from build123d import *

# Parameters (mm, degrees)
F0_R      = 4.925
F1_DEPTH  = 1.55
F2_W      = 1.55
F2_H      = 68.6
F3_DEPTH  = 16
F4_W      = 47.8
F4_H      = 1.55
F5_DEPTH  = 1.55
F6_W      = 47.8
F6_H      = 1.55
F7_DEPTH  = 34.2
F8_R      = 1.5
F10_DEPTH = 1.551


with BuildPart() as f1:
    # F0 (on Top) → F1 (new body)
    with BuildSketch(Plane.XY):
        Polygon((-51.3558513849, 10.4234758295), (-51.3558513849, -58.2765241705), (2.4441486151, -58.2765241705), (2.4441486151, -29.3765241705), (-37.3558513849, 10.4234758295), align=None)
        with BuildLine():
            ThreePointArc((-27.6816260073, -49.4227633754), (-35.7418681063, -49.3109720316), (-35.6300767624, -41.2507299325))
            Line((-35.6300767624, -41.2507299325), (-20.1462239232, -26.190507449))
            ThreePointArc((-20.1462239232, -26.190507449), (-13.9542389387, -25.0256630672), (-10.4719985456, -30.2765241705))
            ThreePointArc((-10.4719985456, -30.2765241705), (-10.9211374423, -32.4942837773), (-12.197773168, -34.3625408919))
            Line((-12.197773168, -34.3625408919), (-27.6816260073, -49.4227633754))
        make_face(mode=Mode.SUBTRACT)
        with Locations((-31.2308513849, -20.5015241705)):
            Circle(F0_R, mode=Mode.SUBTRACT)
    extrude(amount=F1_DEPTH)

    # F2 (on face) → F3 (join)
    with BuildSketch(Plane(origin=(0, 0, 0), x_dir=(1, 0, 0), z_dir=(0, 0, -1))):
        with Locations((-50.5808513849, 23.8765241705)):
            Rectangle(F2_W, F2_H)
    extrude(amount=F3_DEPTH)

    # F4 (on face) → F5 (join)
    with BuildSketch(Plane.XY.offset(1.55)):
        with Locations((-21.4558513849, -59.0515241705)):
            Rectangle(F4_W, F4_H)
    extrude(amount=-F5_DEPTH)

    # F6 (on face) → F7 (join)
    with BuildSketch(Plane.XY.offset(1.55)):
        with Locations((-21.4558513849, -59.0515241705)):
            Rectangle(F6_W, F6_H)
    extrude(amount=F7_DEPTH)

    # F8
    f8_edges = [f1.edges().sort_by_distance(p)[0] for p in [
        (-21.455851, -59.826524, 0),
        (-51.355851, -23.926524, 1.55),
    ]]
    fillet(f8_edges, radius=F8_R)

    # F9 (on face) → F10 (cut, through all)
    with BuildSketch(Plane(origin=(0, -58.2765241705, 0), x_dir=(-1, 0, 0), z_dir=(0, 1, 0))):
        with BuildLine():
            ThreePointArc((15.4058513849, 15.85), (19.3302940204, 17.4755573644), (20.9558513849, 21.4))
            ThreePointArc((20.9558513849, 21.4), (19.3302940204, 25.3244426356), (15.4058513849, 26.95))
            ThreePointArc((15.4058513849, 26.95), (9.8558513849, 21.4), (15.4058513849, 15.85))
        make_face()
        with BuildLine():
            ThreePointArc((15.4058513849, 26.95), (19.3302940204, 25.3244426356), (20.9558513849, 21.4))
            ThreePointArc((20.9558513849, 21.4), (19.3302940204, 17.4755573644), (15.4058513849, 15.85))
            Line((15.4058513849, 15.85), (29.6058513849, 15.85))
            ThreePointArc((29.6058513849, 15.85), (24.0558513849, 21.4), (29.6058513849, 26.95))
            Line((29.6058513849, 26.95), (15.4058513849, 26.95))
        make_face()
        with BuildLine():
            ThreePointArc((35.1558513849, 21.4), (33.5302940204, 25.3244426356), (29.6058513849, 26.95))
            ThreePointArc((29.6058513849, 26.95), (24.0558513849, 21.4), (29.6058513849, 15.85))
            ThreePointArc((29.6058513849, 15.85), (33.5302940204, 17.4755573644), (35.1558513849, 21.4))
        make_face()
    extrude(amount=-F10_DEPTH, mode=Mode.SUBTRACT)


solid = f1.part
Geometry: final body of the model. Coordinates: model frame, mm. A direction names the side the tool comes from. Coordinates: 2 decimals unless noted, no trailing zeros. Order: outer loops, then holes, each group sorted by start corner. A loop starts at its lowest first (then second) coordinate and runs counter-clockwise, first axis right, second up.
(1) Section query A-A (y = -45.5). Return the cut outline in (x, z).
(2) Section query B-B (x = -32). Return the cut outline in (y, z), plus the area to 3 significant figures.
(3) Section query D-D (x = -3.5). Return the cut outline in (y, z).
(4) Access query for faces 1 (the face through (-48, -58.277, 1)), 2 (the face through (-22, -58.277, 15)), 3 (the face through (-51, -58.177, -8)), 4 (the face through (-9.857, -59.041, 21.522)). Directions: +Z, -Z, +X, -X, +Y, -Y. A direction counts if a zero-diameter tool reaches every point of the face in a straight line with its end or side. Return the directions, or none.
(5) Section query C-C (y = -14). Return the cut outline in (x, z).
(6) Draft query along X for faces 5 (the face through (-51.356, -23, -8)), 6 (the face through (-50, 10.423, -4)), 7 (the face through (-49.806, -23, -8)), 8 (the face through (-28, -33.83, 0.76)). Return one class per face: pulls with the +X half, pulls with the -X half, needs draft (parallel to the pull), parting line crosses it, or undercut.
(7) First-contact query: pin 1 (1 mm diameter, centred on x = -39.5, y = -47, fed in from -Z); pin 2 (13 mm diameter, centred on y = -21, z = -8, fed in from +X); pin 3 (12 mm diameter, centred on x = -31.5, z = -5, fed in from -Y); pin 4 (5 mm diameter, centred on x = -32, y = -47.5, fed in from -Z). Flat tips, straight axial feed; report the tip coordinate or a pass-through.
(8) Material intervals for probe 1 along Z at (x, y) = (-47, -14.5); probe 2 along X at (y, z) = (-14.5, -8); probe 3 along Y at (x, z) = (-8, 16), sorted ascending.
Solution:
1. outline: (-51.36, -16) - (-49.81, -16) - (-49.81, 0) - (-37.35, 0) - (-37.35, 1.55) - (-49.86, 1.55) arc R1.5 ccw to (-51.36, 0.05) - close; (-23.65, 0) - (2.44, 0) - (2.44, 1.55) - (-23.65, 1.55) - close
2. outline: (-59.83, 1.5) arc R1.5 ccw to (-58.33, 0) - (-51.03, 0) - (-51.03, 1.55) - (-58.28, 1.55) - (-58.28, 16.39) - (-59.83, 16.39) - close; (-59.83, 26.41) - (-58.28, 26.41) - (-58.28, 35.75) - (-59.83, 35.75) - close; (-37.72, 0) - (-25.37, 0) - (-25.37, 1.55) - (-37.72, 1.55) - close; (-15.64, 0) - (5.07, 0) - (5.07, 1.55) - (-15.64, 1.55) - close
2. area: 102 mm2
3. outline: (-59.83, 1.5) arc R1.5 ccw to (-58.33, 0) - (-23.43, 0) - (-23.43, 1.55) - (-58.28, 1.55) - (-58.28, 35.75) - (-59.83, 35.75) - close
4. face 1: +Z, -Z, -X, -Y
4. face 2: +Z, +X, -X, +Y
4. face 3: -Z, +X, -X, -Y
4. face 4: +Y, -Y
5. outline: (-51.36, -16) - (-49.81, -16) - (-49.81, 0) - (-12.93, 0) - (-12.93, 1.55) - (-49.86, 1.55) arc R1.5 ccw to (-51.36, 0.05) - close
6. face 5: pulls with the -X half
6. face 6: needs draft
6. face 7: pulls with the +X half
6. face 8: undercut
7. pin 1: stops at z = 0
7. pin 2: stops at x = -49.81
7. pin 3: stops at y = -59.74
7. pin 4: passes through
8. probe 1: z = 0 to 1.55
8. probe 2: x = -51.36 to -49.81
8. probe 3: y = -59.83 to -58.28
